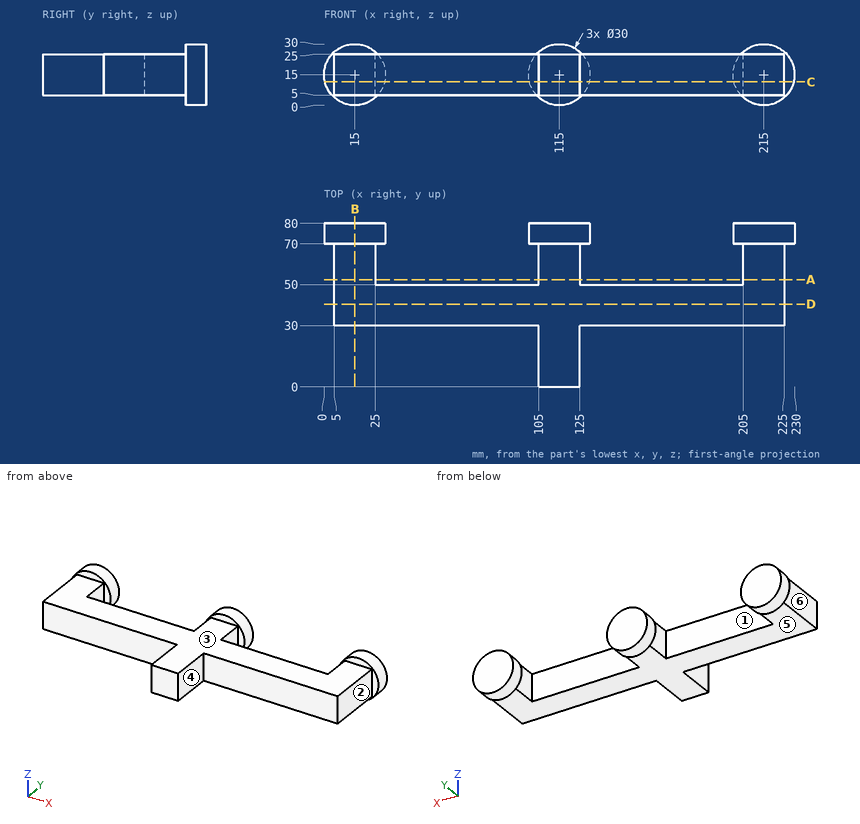
Study the drawing (mm; zero at the part's minimum x, y, z) and answer. A direction names the side the tool comes from. Coordinates: 2 decimals unless noted, no trailing zeros. Write each loop counter-clockwise with the first axis right and the second up, starting at its lowest first coordinate (ties: lowest second). Pieces come first, ordered by that corner, then holes. Notation, with made-up numbers: M 71.25,-10.75 L 113.25,-10.75 A20 cw 113.25,28.25 Z; hole C -21,80 d6. An arc over 180 degrees is marked long. Use a Markdown table: item, result. Add a question column.
1. Section B-B (x = 15) is taken. Give the vertices of the cut face in (y, z), plus the area to 3 significant figures.
2. Section A-A (y = 52.5) is taken. Give the vertices of the cut face in (x, z).
3. Section C-C (z = 11.5) is taken. Give the vertices of the cut face in (x, y), plus the area to 3 significant figures.
4. For a pull along X with two mould halves and no side action, classify the marked faces 1, 2 and 3 as +X half, -X half, draft (parallel to the pull), parting line (faces both ways), or undercut.
5. Straight lines are drawn through the part: line 1 along X through (y, z) = (63, 21.75); line 2 along X through (y, z) = (70.5, 15.25); line 3 along X through (y, z) = (9.5, 18). For each, find the intervals that lie inside material, in ascending order. Write a range as [from, to].
6. Section D-D (y = 40.5) is taken. Give the vertices of the cut face in (x, z), plus the area to 3 significant figures.
7. Given P1, Ø4, axis at x = 48.5, z = 21, coming from the +Y side; P2, Ø16, axis at y = 61, z = 20, coming from the -X side; P3, Ø6, axis at y = 10, z = 17.5, coming from the +X side, each flat-ended and moving along its own axis, determine where each tip first touches the part or whether it passes through.
8. Which of the six approach directions +Z, -Z, +X, -X, +Y, -Y give full straight-line access (tool end or side, diameter ignored) to the marked faces 4, 5 and 6?
Data:
| question | item | result |
|---|---|---|
| 1 | outline | M 30,5 L 70,5 L 70,0 L 80,0 L 80,30 L 70,30 L 70,25 L 30,25 Z |
| 1 | area | 1,100 mm2 |
| 2 | outline | M 5,5 L 25,5 L 25,25 L 5,25 Z; M 105,5 L 125,5 L 125,25 L 105,25 Z; M 205,5 L 225,5 L 225,25 L 205,25 Z |
| 3 | outline | M 0.41,70 L 5,70 L 5,30 L 105,30 L 105,0 L 125,0 L 125,30 L 225,30 L 225,70 L 229.59,70 L 229.59,80 L 200.41,80 L 200.41,70 L 205,70 L 205,50 L 125,50 L 125,70 L 129.59,70 L 129.59,80 L 100.41,80 L 100.41,70 L 105,70 L 105,50 L 25,50 L 25,70 L 29.59,70 L 29.59,80 L 0.41,80 Z |
| 3 | area | 7,080 mm2 |
| 4 | face 1 | undercut |
| 4 | face 2 | +X half |
| 4 | face 3 | draft |
| 5 | line 1 | x = [5, 25], [105, 125], [205, 225] |
| 5 | line 2 | x = [0, 30], [100, 130], [200, 230] |
| 5 | line 3 | x = [105, 125] |
| 6 | outline | M 5,5 L 225,5 L 225,25 L 5,25 Z |
| 6 | area | 4,400 mm2 |
| 7 | P1 | stops at y = 50 |
| 7 | P2 | stops at x = 5 |
| 7 | P3 | stops at x = 125 |
| 8 | face 4 | +Z, -Z, +X, -Y |
| 8 | face 5 | -Z, +X, -X, -Y |
| 8 | face 6 | +Z, -Z, -X, -Y |
